Autodesk Inventor part; units mm, degrees
ref_plane "YZ Plane" through (0, 0, 0) normal (1, 0, 0) x (0, 1, 0)
ref_plane "XZ Plane" through (0, 0, 0) normal (0, 1, 0) x (-1, 0, 0)
ref_plane "XY Plane" through (0, 0, 0) normal (0, 0, 1) x (1, 0, 0)
sketch "Sketch_13" plane through (0, 0, 0) normal (0, 0, 1) x (1, 0, 0)
  line L0 (2, 0) -> (-2, 0)
  arc A0 (0, 2.15) -> (0.15, 2) centre (0.15, 2.15) ccw
  line L1 (0.15, 2) -> (3.85, 2)
  arc A1 (3.85, 2) -> (4, 2.15) centre (3.85, 2.15) ccw
  line L2 (4, 2.15) -> (4, 2.95)
  line L3 (4, 2.95) -> (2.52, 2.95)
  arc A2 (1.48, 2.95) -> (2.52, 2.95) centre (2, 3.55) ccw
  line L4 (1.48, 2.95) -> (0, 2.95)
  line L5 (0, 2.95) -> (0, 2.15)
revolve "Revolution1" add sketch "Sketch_13" angle 360 about axis through (2, 0, 0) along (1, 0, 0)
sketch "Sketch_25" plane through (0, 0, 0) normal (0, 0, 1) x (1, 0, 0)
  line L0 (50, 0) -> (-50, 0)
  line L1 (0.0375, 4.4) -> (0.06, 4.0375)
  line L2 (0.06, 4.0375) -> (0.0375, 3.675)
  line L3 (0.0375, 3.675) -> (0.0375, 2.95)
  line L4 (0.0375, 2.95) -> (0.0825, 2.95)
  line L5 (0.0825, 2.95) -> (0.1275, 3.675)
  line L6 (0.1275, 3.675) -> (0.1275, 4.0375)
  line L7 (0.1275, 4.0375) -> (0.0825, 4.4)
  line L8 (0.0825, 4.4) -> (0.0375, 4.4)
revolve "Revolution2" add sketch "Sketch_25" angle 360 about axis through (50, 0, 0) along (1, 0, 0)
sketch "Sketch_26" plane through (0, 0, 0) normal (0, 0, 1) x (1, 0, 0)
  line L0 (50, 0) -> (-50, 0)
  line L1 (3.8725, 4.0375) -> (3.8725, 3.675)
  line L2 (3.8725, 3.675) -> (3.9175, 2.95)
  line L3 (3.9175, 2.95) -> (3.9625, 2.95)
  line L4 (3.9625, 2.95) -> (3.9625, 3.675)
  line L5 (3.9625, 3.675) -> (3.94, 4.0375)
  line L6 (3.94, 4.0375) -> (3.9625, 4.4)
  line L7 (3.9625, 4.4) -> (3.9175, 4.4)
  line L8 (3.9175, 4.4) -> (3.8725, 4.0375)
revolve "Revolution3" add sketch "Sketch_26" angle 360 about axis through (50, 0, 0) along (1, 0, 0)
properties part number "W 638/4 XR-2Z_PART1"
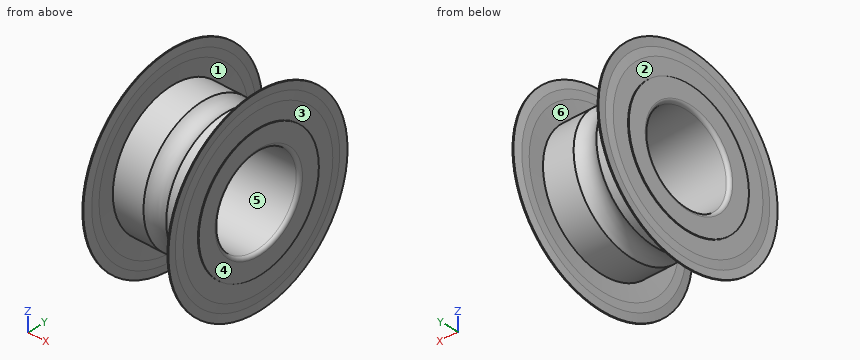
Could you check a few things on this model? Use its own coordinates, in mm. Face numbers are marked on the shaded views. A direction names the side the tool comes from. Round coordinates to 2 decimals unless told otherwise and drop trailing zeros. Write each loop counter-clockwise with the first axis right and the second up, starting at its lowest first coordinate (ties: lowest second). Pieces come first, ordered by that corner, then holes. Notation, with made-up numbers: (40, -9) -> (54, -9) arc R14 cw to (54, 13) -> close; hole circle Ø7 at (40.25, 67.5). An arc over 180 degrees is marked (long way). Use a Markdown table: item, result.
1. We'd pull the mould along Z, two halves only. Please class the marked faces 4, 5 and 6: +Z half, -Z half, draft (parallel to the pull), parting line (faces both ways), or undercut.
Answer key:
| item | result |
|---|---|
| face 4 | draft |
| face 5 | undercut |
| face 6 | undercut |
2. Which directions (+Z, -Z, +X, -X, +Y, -Y) give clear straight access to the entire face, cutting with the end or side of a thin tool? Please do the marked faces 1, 2 and 3.
Answer key:
| item | result |
|---|---|
| face 1 | none |
| face 2 | -X |
| face 3 | +X |
3. If we section it at A-A (x = 3.2): List the corners of the cut face in (y, z) for me, then the cut area to 3 significant figures.
Answer key:
| item | result |
|---|---|
| outline | circle Ø5.9 at (0, 0); hole circle Ø4 at (0, 0) |
| area | 14.8 mm^2 |
4. If we section it at B-B (x = 2): List the corners of the cut face in (y, z) for me.
Answer key:
| item | result |
|---|---|
| outline | circle Ø5.51 at (0, 0); hole circle Ø4 at (0, 0) |
5. For pin 1 Ø1.5 at (y, z) = (3, 2.5) entering from +X, with a flat end and sliding along its axis, tell me the tip position at first contact or that it passes through.
Answer key:
| item | result |
|---|---|
| pin 1 | stops at x = 3.96 |
6. Please list where these lines run through material, in increasing order: probe 1 along Z at (x, y) = (2.65, 0); probe 2 along Y at (x, z) = (0.4, 1.5); probe 3 along Y at (x, z) = (2.5, -1).
Answer key:
| item | result |
|---|---|
| probe 1 | z = -2.95 to -2, 2 to 2.95 |
| probe 2 | y = -2.54 to -1.32, 1.32 to 2.54 |
| probe 3 | y = -2.76 to -1.73, 1.73 to 2.76 |
